Here's how the part is built. I have some questions about the finished solid (model axes, mm). Face numbers are marked on the shaded views. A direction names the side the tool comes from. Give positions to 0.01 mm unless a question says otherwise; leave off trailing zeros. Order: outer loops, then holes, each group sorted by start corner. A loop starts at its lowest first (then second) coordinate and runs counter-clockwise, first axis right, second up. Notation, with made-up numbers: (15.25, -23) -> (74.25, -23) arc R14 cw to (74.25, -5) -> close; hole circle Ø7 at (87, 19.5). An arc over 180 degrees is marked (long way). Write each question's results on one line, items separated by ' | '. Start each with the question number.
Q1. For the marked faces 1 and 2, which set-ups out of +Z, -Z, +X, -X, +Y, -Y let a thin tool reach every point of the face, with its end or its side?
Q2. Imagine slicing it at C-C, the plane y = -10. Please give me the cut outline in (x, z), then the cut area to 3 significant figures.
Q3. Imagine slicing it at D-D, the plane x = 8. Please give me the cut outline in (y, z).
Q4. I need wall thicknesses on line 1 along Y through (x, z) = (43, 232); line 2 along Y through (x, z) = (26, 121); line 3 along X through (y, z) = (22, 202). Which ranges of each line are inside material? Lowest first, please. Write a range as [from, to].
Q5. Imagine slicing it at A-A, the plane x = 37. Please give me the cut outline in (y, z).
Q6. Thinking about a two-plate mould opening in Y: for the marked faces 3, 4, 5 and 6, which applies, pulls with the +Y half, pulls with the -Y half, needs draft (parallel to the pull), parting line crosses it, or undercut?
Q7. I'm going to push a flat-ended pin straight in: pin 1 (12 mm diameter, centred on y = 13.5, z = 105, fed in from +X). Where does the tip first touch, or does it pass through?
Q8. Imagine slicing it at B-B, the plane z = 221.5. Please give me the cut outline in (x, y), then the cut area to 3 significant figures.
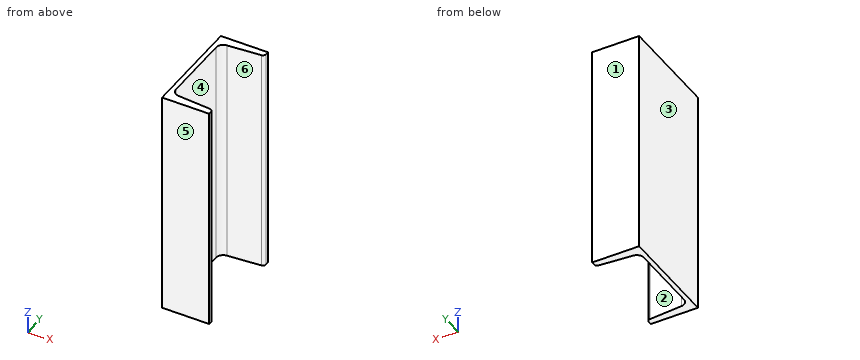
Autodesk Inventor part; units mm, degrees
ref_plane "Начальная плоскость" through (0, 0, 23) normal (0, 0, 1) x (1, 0, 0)
ref_plane "Конечная плоскость" through (0, 0, 246) normal (0, 0, 1) x (1, 0, 0)
ref_plane "РабПлоскость8" through (169.5, -50, 246) normal (0, 0, 1) x (1, 0, 0)
ref_plane "Начальная плоскость" through (0, 0, 23) normal (0, 0, 1) x (1, 0, 0)
ref_plane "Конечная плоскость" through (0, 0, 246) normal (0, 0, 1) x (1, 0, 0)
sketch "Эскиз" plane through (0, 0, 0) normal (0, 0, 1) x (1, 0, 0)
  line L0 (46, -50) -> (0, -50)
  line L1 (46, -50) -> (46, -46.6496)
  line L2 (43.2392, -43.6591) -> (10.9418, -41.0753)
  line L3 (4.5, -34.0976) -> (4.5, 34.0976)
  line L4 (43.2392, 43.6591) -> (10.9418, 41.0753)
  line L5 (46, 46.6496) -> (46, 50)
  line L6 (0, 50) -> (46, 50)
  line L7 (0, -50) -> (0, 50)
  arc A0 (4.5, -34.0976) -> (10.9418, -41.0753) centre (11.5, -34.0976) ccw
  arc A1 (10.9418, 41.0753) -> (4.5, 34.0976) centre (11.5, 34.0976) ccw
  arc A2 (46, -46.6496) -> (43.2392, -43.6591) centre (43, -46.6496) ccw
  arc A3 (43.2392, 43.6591) -> (46, 46.6496) centre (43, 46.6496) ccw
  line L8 (0, 70) -> (0, -70) construction
  line L9 (-9.3169, 0) -> (55.9016, 0) construction
  point P0 (46, -43.88)
  point P1 (4.5, -40.56)
  point P2 (4.5, 40.56)
  point P3 (46, 43.88)
  dimension "d3" = 46
  dimension "d5" = 4.5
  dimension "d7" = 100
  dimension "d9" = 9.44
  dimension "d11" = 9.44
  dimension "d13" = 6.12
  dimension "d15" = 6.12
  dimension "d22" = 7
  dimension "d23" = 3
  dimension "d24" = 50
  dimension "d25" = 0
extrude "Тело" add sketch "Эскиз" along normal up to surface (223 mm away) from surface at 23
sketch "Sketch3" plane through (0, 0, 0) normal (0, 0, 1) x (1, 0, 0)
  line L0 (0, 0) -> (10, 0)
ref_plane "Work Plane7" through (0, 0, 0) normal (0, -1, 0) x (1, 0, 0)
sketch "Sketch4" plane through (0, 0, 0) normal (0, -1, 0) x (1, 0, 0)
  line L0 (-2, 23) -> (12, 23)
  line L1 (-2, 246) -> (12, 246)
  dimension "d29" = 223
ref_plane "РабПлоскость8" through (169.5, -50, 246) normal (0, 0, 1) x (1, 0, 0)
split "Разделение1" plane through (169.5, -50, 246) removes the side toward (0, 0, 1)
ref_plane "РабПлоскость9" through (-479.5, -50, 23) normal (0, 0, -1) x (-1, 0, 0)
split "Разделение2" plane through (-479.5, -50, 23) removes the side toward (0, 0, -1)
equation "\"d3\" = b"
equation "\"d7\" = ParH"
equation "\"d22\" = R"
equation "\"d23\" = R1"
equation "\"d24\" = 0.5 * d7"
equation "\"d16\" = G_L"
equation "\"R1\" = 3"
equation "\"R\" = 7"
equation "\"t1\" = 4.5"
equation "\"t2\" = 7.6"
equation "\"ParH\" = 100"
equation "\"b\" = 46"
equation "\"msp_x1\" = 0.04 * b"
equation "\"msp_x2\" = -0.08 * t1 + 0.04 * b"
equation "\"G_L\" = d29"
equation "\"ex\" = 0"
equation "\"G_OFFSET_START\" = -23"
equation "\"G_OFFSET_END\" = -23"
equation "\"d26\" = -G_OFFSET_START"
equation "\"d27\" = G_OFFSET_END + B_L"
equation "\"B_L\" = 269"
properties part number "Швеллер 10U-223 ГОСТ 8240-97" material "Сталь, мягкая"
Geometry check:
1) face 1: +Z, -Z, +X, -X, +Y | face 2: +Z, -Z, +X
2) outline: (0, 23) -> (4.5, 23) -> (4.5, 246) -> (0, 246) -> close | area: 1,000 mm²
3) outline: (-50, 23) -> (-40.16, 23) -> (-40.16, 246) -> (-50, 246) -> close; (40.16, 23) -> (50, 23) -> (50, 246) -> (40.16, 246) -> close
4) line 1: [-50, -43.64], [43.64, 50] | line 2: [-50, -42.28], [42.28, 50] | line 3: [0, 4.5]
5) outline: (-50, 23) -> (-43.16, 23) -> (-43.16, 246) -> (-50, 246) -> close; (43.16, 23) -> (50, 23) -> (50, 246) -> (43.16, 246) -> close
6) face 3: needs draft | face 4: undercut | face 5: pulls with the -Y half | face 6: undercut
7) pin 1: x = 4.5
8) outline: (0, -50) -> (46, -50) -> (46, -46.65) arc R3 ccw to (43.24, -43.66) -> (10.94, -41.08) arc R7 cw to (4.5, -34.1) -> (4.5, 34.1) arc R7 cw to (10.94, 41.08) -> (43.24, 43.66) arc R3 ccw to (46, 46.65) -> (46, 50) -> (0, 50) -> close | area: 1,110 mm²
